Part print with two shaded views. Sizes in mm from the minimum x, y, z corner. A direction names the side the tool comes from. Round coordinates to 2 decimals unless told otherwise and drop trailing zeros. Order: outer loops, then holes, each group sorted by start corner. A loop starts at its lowest first (then second) coordinate and runs counter-clockwise, first axis right, second up. Notation, with made-up numbers: M 29,24 L 34,24 A17 cw 34,31 Z; hole C 19.5,9 d3. An arc over 180 degrees is marked long. Answer as a JSON object with one key per item and string values.
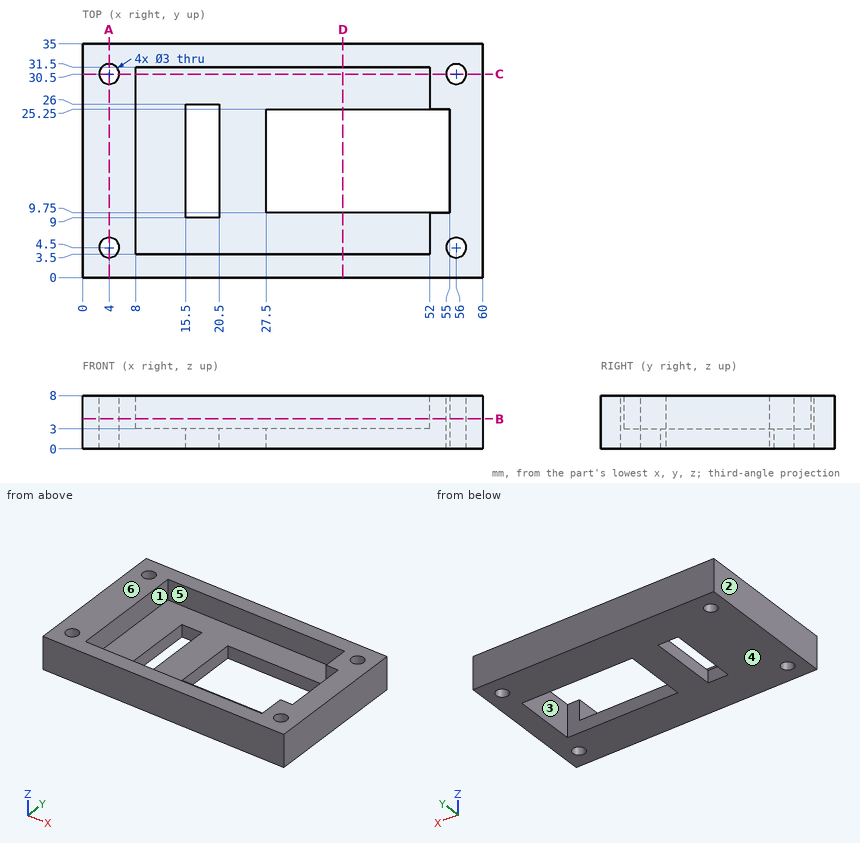
Item 1: 3-axis set-ups, long thin cutter, end or side, ignore diameter. For the marked faces 5 and 6: which of +Z, -Z, +X, -X, +Y, -Y reach the whole face in a straight line?
Worked answers:
{"face 5": "+Z", "face 6": "+Z, +X, -X, +Y, -Y"}
Item 2: Saw through at A-A on x = 4. List the corners of the cut face in (y, z), and give its area (3 significant figures).
Worked answers:
{"outline": "M 0,0 L 3,0 L 3,8 L 0,8 Z; M 6,0 L 29,0 L 29,8 L 6,8 Z; M 32,0 L 35,0 L 35,8 L 32,8 Z", "area": "232 mm2"}
Item 3: Saw through at C-C on y = 30.5. List the corners of the cut face in (x, z).
Worked answers:
{"outline": "M 0,0 L 2.5,0 L 2.5,8 L 0,8 Z; M 5.5,0 L 54.5,0 L 54.5,8 L 52,8 L 52,3 L 8,3 L 8,8 L 5.5,8 Z; M 57.5,0 L 60,0 L 60,8 L 57.5,8 Z"}
Item 4: Drop flat-ended pins along their axis: pin 1 Ø5 at (x, y) = (4, 4.5) entering from -Z; pin 2 Ø8.5 at (x, y) = (19.5, 18) entering from +Z. Give the stop position or say it passes through.
Worked answers:
{"pin 1": "stops at z = 0", "pin 2": "stops at z = 3"}
Item 5: Saw through at D-D on x = 39. List the corners of the cut face in (y, z).
Worked answers:
{"outline": "M 0,0 L 9.75,0 L 9.75,3 L 3.5,3 L 3.5,8 L 0,8 Z; M 25.25,0 L 35,0 L 35,8 L 31.5,8 L 31.5,3 L 25.25,3 Z"}
Item 6: Wall check: line 1 along X through (y, z) = (22.5, 2); line 2 along X through (y, z) = (30.5, 7); line 3 along X through (y, z) = (4.5, 1.5). Give the ranges that are in metal, low to high. Write a range as [from, to].
Worked answers:
{"line 1": "x = [0, 15.5], [20.5, 27.5], [55, 60]", "line 2": "x = [0, 2.5], [5.5, 8], [52, 54.5], [57.5, 60]", "line 3": "x = [0, 2.5], [5.5, 54.5], [57.5, 60]"}
Item 7: Two-plate mould, pull along X, no slides. Class the marked faces 1, 2, 3 and 4: released by +X, released by -X, zero draft, split by the parting line, or undercut.
Worked answers:
{"face 1": "undercut", "face 2": "released by -X", "face 3": "undercut", "face 4": "zero draft"}
Item 8: Saw through at B-B on z = 4.5. List the corners of the cut face in (x, y).
Worked answers:
{"outline": "M 0,0 L 60,0 L 60,35 L 0,35 Z; hole C 4,4.5 d3; hole C 4,30.5 d3; hole M 8,3.5 L 52,3.5 L 52,9.75 L 55,9.75 L 55,25.25 L 52,25.25 L 52,31.5 L 8,31.5 Z; hole C 56,4.5 d3; hole C 56,30.5 d3"}
